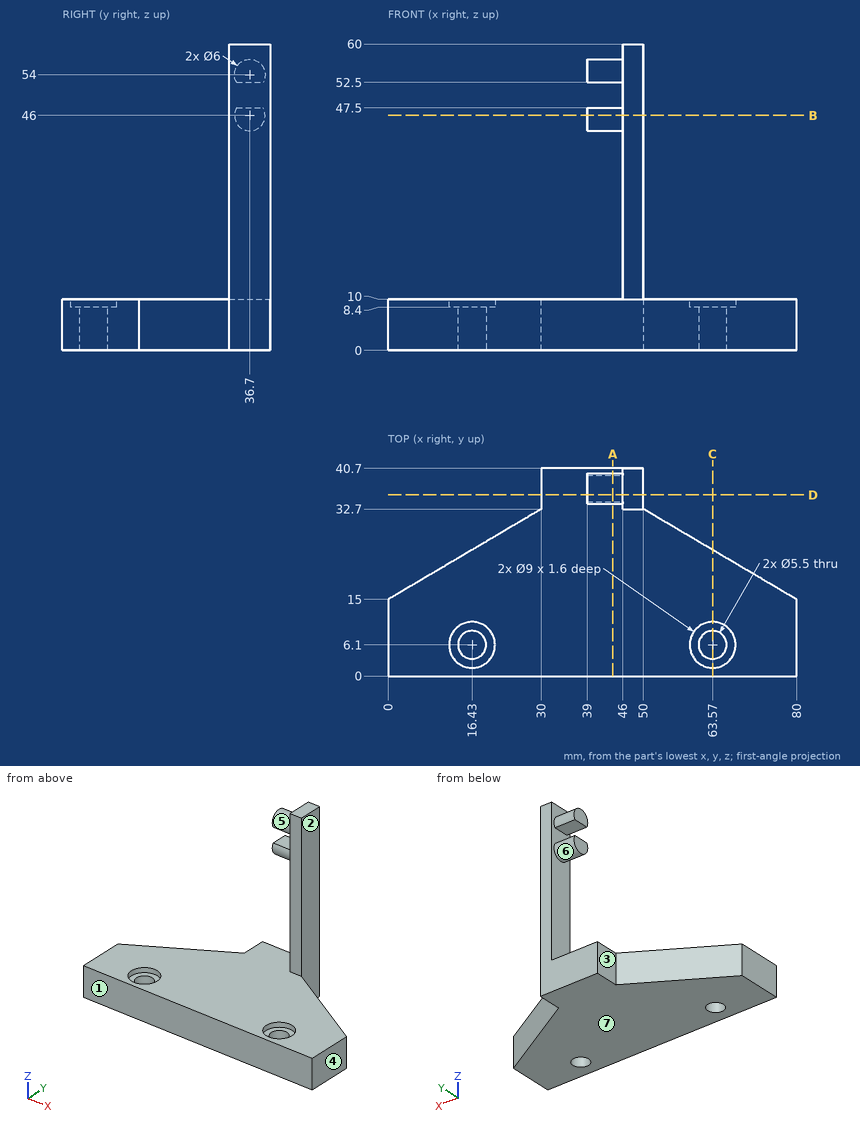
The figure shows three views and two pictorial views of one solid part (mm, origin at its lowest corner). Answer the questions. A direction names the side the tool comes from. Give positions to 0.01 mm unless a question says otherwise; leave off trailing zeros. Write each loop counter-clockwise with the first axis right and the second up, starting at its lowest first coordinate (ties: lowest second). Pieces come first, ordered by that corner, then holes. Notation, with made-up numbers: (87.25, 8.25) -> (123.25, 8.25) arc R26 ccw to (123.25, 36.25) -> close; hole circle Ø7 at (87.5, 51). An arc over 180 degrees is marked (long way). Write each question's results on one line, items separated by ' | '.
1. A tool of negligible diameter and unlimited length cuts with its end or side. For the marked faces 1, 2 and 3, from which of +Z, -Z, +X, -X, +Y, -Y can it reach the whole face along a straight path? Write none if from no direction.
Data:
face 1: +Z, -Z, +X, -X, -Y | face 2: +Z, -Z, +X, +Y | face 3: +Z, -Z, -X, +Y
2. Find section B-B on z = 46. Determine the outline of the cut face in (x, y), and give its area (3 significant figures).
Data:
outline: (39, 33.7) -> (46, 33.7) -> (46, 32.7) -> (50, 32.7) -> (50, 40.7) -> (46, 40.7) -> (46, 39.7) -> (39, 39.7) -> close | area: 74.0 mm^2
3. Each of these flat-tipped pins is pushed along its axis until it touches: pin 1 Ø2.5 at (x, y) = (16.5, 8) entering from +Z; pin 2 Ø4 at (x, y) = (10, 21) entering from -Z; pin 3 Ø1.3 at (y, z) = (37, 54.5) entering from -X; pin 4 Ø2.5 at (y, z) = (35, 34) entering from +X. Where does it stop, or does it pass through?
Data:
pin 1: z = 8.4 | pin 2: z = 0 | pin 3: x = 39 | pin 4: x = 50
4. Find section C-C on x = 63.57. Determine the outline of the cut face in (y, z), and give its area (3 significant figures).
Data:
outline: (0, 0) -> (3.35, 0) -> (3.35, 8.4) -> (1.6, 8.4) -> (1.6, 10) -> (0, 10) -> close; (8.85, 0) -> (24.69, 0) -> (24.69, 10) -> (10.6, 10) -> (10.6, 8.4) -> (8.85, 8.4) -> close | area: 186 mm^2
5. Determine the mould class of the marked faces 4, 5, 6 and 7 for opening direction Z: +Z half, -Z half, draft (parallel to the pull), parting line (faces both ways), or undercut.
Data:
face 4: draft | face 5: undercut | face 6: undercut | face 7: -Z half
6. Find section D-D on y = 35.5. Determine the outline of the cut face in (x, z).
Data:
outline: (30, 0) -> (50, 0) -> (50, 60) -> (46, 60) -> (46, 56.75) -> (39, 56.75) -> (39, 52.5) -> (46, 52.5) -> (46, 47.5) -> (39, 47.5) -> (39, 43.25) -> (46, 43.25) -> (46, 10) -> (30, 10) -> close
7. Straight lines are drawn through the part: L1, parallel to X at y = 6, z = 8; L2, parallel to Z at x = 34.5, y = 35; L3, parallel to X at y = 8.5, z = 6.5. For each, find the intervals that lie inside material, in ascending order.
Data:
L1: 0 to 13.68, 19.18 to 60.82, 66.32 to 80 | L2: 0 to 10 | L3: 0 to 15.09, 17.77 to 62.23, 64.91 to 80
8. Find section A-A on x = 44. Determine the outline of the cut face in (y, z).
Data:
outline: (0, 0) -> (40.7, 0) -> (40.7, 10) -> (0, 10) -> close; (34.1, 47.5) arc R3 ccw (long way) to (39.3, 47.5) -> close; (34.1, 52.5) -> (39.3, 52.5) arc R3 ccw (long way) to start
